Verification items for the finished model (mm, model axes). Face numbers are marked on the shaded views. A direction names the side the tool comes from. Round coordinates to 2 decimals unless told otherwise and drop trailing zeros. Order: outer loops, then holes, each group sorted by start corner. A loop starts at its lowest first (then second) coordinate and runs counter-clockwise, first axis right, second up. Notation, with made-up numbers: (75, 15) -> (122, 15) arc R18 ccw to (122, 39) -> close; hole circle Ø2 at (2, 86.25). An arc over 180 degrees is marked (long way). Return JSON: item names as keys, results as strings. Group by question number.
1) Section check D-D on z = 9. Enter the section's corners in (x, y).
2) Section check A-A on z = 24. Enter the section's corners in (x, y).
3) Section check C-C on y = 20. Enter the section's corners in (x, z), plus the area to 3 significant figures.
4) Tool access check on the marked faces 1 and 2. Record the directions out of +Z, -Z, +X, -X, +Y, -Y that give a thin tool (end or side, any length) a straight path to the whole face; none if there is none.
5) Depth check by flat-ended pin: pin 1 (1 mm diameter, centred on x = -39, y = 18.5, fed in from +Z); pin 2 (7.5 mm diameter, centred on x = -18, y = 40, fed in from -Z); pin 3 (4 mm diameter, centred on x = -7, y = 40, fed in from -Z). Enter the tip coordinate at first touch or a pass-through.
6) Scan lines: L1, parallel to Y at x = -18, z = 3.05; L2, parallel to X at y = 2.5, z = 30.5; L3, parallel to Z at x = -60, y = 13.5. Record each from-to range of solid material in increasing order.
7) Section check B-B on x = -7. Enter the section's corners in (y, z).
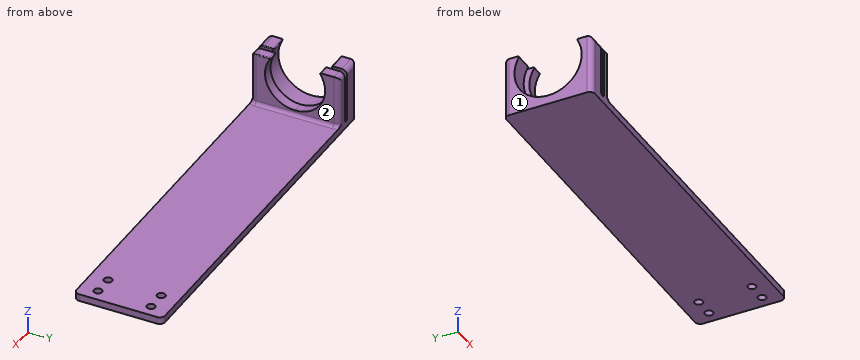
```python
from build123d import *

# Parameters (mm, degrees)
SKETCH_1_W                      = 210
SKETCH_1_H                      = 50
EXTRUDE_1_DEPTH                 = 4
CUT_EXTRUDE_1_REACH             = 217.907
SKETCH_4_R                      = 2.3
CUT_EXTRUDE_1_DIRECTION_2_DEPTH = 216.907387553
EXTRUDE_2_DEPTH                 = 10
EXTRUDE_3_DEPTH                 = 6
FILLET_1_R                      = 3
FILLET_2_R                      = 2
FILLET_3_R                      = 1
FILLET_4_R                      = 0.5


# Some blends are built 0.0001 mm under size
with BuildPart() as part:
    # ｽｹｯﾁ1 → ﾎﾞｽ - 押し出し1 (new body)
    with BuildSketch(Plane.XY):
        with Locations((-105, 25)):
            Rectangle(SKETCH_1_W, SKETCH_1_H)
    extrude(amount=EXTRUDE_1_DEPTH)

    # ｽｹｯﾁ4 → ｶｯﾄ - 押し出し1 (cut, up to next)
    with BuildSketch(Plane.XY.offset(4), mode=Mode.PRIVATE) as cut_extrude_1_sk1:
        with Locations(Location((-7, 40, 0), (0, 0, 180))):
            Circle(SKETCH_4_R)
    cut_extrude_1_tool1 = extrude(cut_extrude_1_sk1.sketch, amount=-CUT_EXTRUDE_1_REACH, mode=Mode.PRIVATE) & part.part
    # ｽｹｯﾁ4 → ｶｯﾄ - 押し出し1 (cut, up to next)
    with BuildSketch(Plane.XY.offset(4), mode=Mode.PRIVATE) as cut_extrude_1_sk2:
        with Locations(Location((-18, 40, 0), (0, 0, 180))):
            Circle(SKETCH_4_R)
    cut_extrude_1_tool2 = extrude(cut_extrude_1_sk2.sketch, amount=-CUT_EXTRUDE_1_REACH, mode=Mode.PRIVATE) & part.part
    # ｽｹｯﾁ4 → ｶｯﾄ - 押し出し1 (cut, up to next)
    with BuildSketch(Plane.XY.offset(4), mode=Mode.PRIVATE) as cut_extrude_1_sk3:
        with Locations(Location((-7, 10, 0), (0, 0, 180))):
            Circle(SKETCH_4_R)
    cut_extrude_1_tool3 = extrude(cut_extrude_1_sk3.sketch, amount=-CUT_EXTRUDE_1_REACH, mode=Mode.PRIVATE) & part.part
    # ｽｹｯﾁ4 → ｶｯﾄ - 押し出し1 (cut, up to next)
    with BuildSketch(Plane.XY.offset(4), mode=Mode.PRIVATE) as cut_extrude_1_sk4:
        with Locations(Location((-18, 10, 0), (0, 0, 180))):
            Circle(SKETCH_4_R)
    cut_extrude_1_tool4 = extrude(cut_extrude_1_sk4.sketch, amount=-CUT_EXTRUDE_1_REACH, mode=Mode.PRIVATE) & part.part
    add(cut_extrude_1_tool1.solids().sort_by_distance((-7, 40, 4))[0], mode=Mode.SUBTRACT)
    add(cut_extrude_1_tool2.solids().sort_by_distance((-18, 40, 4))[0], mode=Mode.SUBTRACT)
    add(cut_extrude_1_tool3.solids().sort_by_distance((-7, 10, 4))[0], mode=Mode.SUBTRACT)
    add(cut_extrude_1_tool4.solids().sort_by_distance((-18, 10, 4))[0], mode=Mode.SUBTRACT)

    # ｽｹｯﾁ4 → ｶｯﾄ - 押し出し1 direction 2 (cut)
    with BuildSketch(Plane.XY.offset(4)):
        with Locations(Location((-7, 40, 0), (0, 0, 180))):
            Circle(SKETCH_4_R)
        with Locations(Location((-18, 40, 0), (0, 0, 180))):
            Circle(SKETCH_4_R)
        with Locations(Location((-7, 10, 0), (0, 0, 180))):
            Circle(SKETCH_4_R)
        with Locations(Location((-18, 10, 0), (0, 0, 180))):
            Circle(SKETCH_4_R)
    extrude(amount=CUT_EXTRUDE_1_DIRECTION_2_DEPTH, mode=Mode.SUBTRACT)

    # ｽｹｯﾁ5 → ﾎﾞｽ - 押し出し2 (add)
    with BuildSketch(Plane.ZY.offset(210)):
        with BuildLine():
            Line((34, 50), (4, 50))
            Line((4, 50), (4, 0))
            Line((4, 0), (34, 0))
            Line((34, 0), (34, 8.844505579))
            ThreePointArc((34, 8.844505579), (5, 25), (34, 41.155494421))
            Line((34, 41.155494421), (34, 50))
        make_face()
    extrude(amount=-EXTRUDE_2_DEPTH)

    # ｽｹｯﾁ6 → ﾎﾞｽ - 押し出し3 (add)
    with BuildSketch(Plane(origin=(-197.7, 0, 0), x_dir=(0, 0, -1), z_dir=(1, 0, 0))):
        with BuildLine():
            Line((-4, 50), (-34, 50))
            Line((-34, 50), (-34, 38.747727085))
            ThreePointArc((-34, 38.747727085), (-16.28637569, 40.149257408), (-7, 25))
            ThreePointArc((-7, 25), (-16.28637569, 9.850742592), (-34, 11.252272915))
            Line((-34, 11.252272915), (-34, 0))
            Line((-34, 0), (-4, 0))
            Line((-4, 0), (-4, 50))
        make_face()
    extrude(amount=EXTRUDE_3_DEPTH)

    # ﾌｨﾚｯﾄ1
    fillet_1_edges = [part.edges().sort_by_distance(p)[0] for p in [
        (-205, 0, 34),
        (-205, 50, 34),
        (-194.7, 0, 34),
        (-191.7, 50, 19),
        (-194.7, 50, 34),
        (-191.7, 0, 19),
        (0, 0, 2),
        (-210, 0, 17),
        (-210, 50, 17),
        (0, 50, 2),
    ]]
    fillet(fillet_1_edges, radius=FILLET_1_R)

    # ﾌｨﾚｯﾄ2
    # the kernel refuses this fillet: 2 mm, written as the material it adds along each edge
    with BuildSketch(Plane(origin=(-191.7, 3, 4), x_dir=(0, 0, 1), z_dir=(0, 1, 0))) as fillet_2_piece_1:
        with BuildLine():
            CenterArc((FILLET_2_R, FILLET_2_R), FILLET_2_R, 180, 90)
            Line((0, FILLET_2_R), (0, 0))
            Line((0, 0), (FILLET_2_R, 0))
        make_face()
    extrude(amount=44)
    with BuildSketch(Plane(origin=(-194.7, 3, 4), x_dir=(-0.9953436464450918, 0.0963899656675329, 0), z_dir=(0.0963899656675329, 0.9953436464450918, 0))) as fillet_2_piece_2_section:
        with BuildLine():
            CenterArc((3 + FILLET_2_R, FILLET_2_R), FILLET_2_R, 180, 90)
            Line((3 + FILLET_2_R, 0), (3, 0))
            Line((3, 0), (3, FILLET_2_R))
        make_face()
    fillet_2_piece_2 = revolve(axis=Axis((-194.7, 3, 4), (0, 0, 1)), revolution_arc=185.531326158, mode=Mode.PRIVATE)
    fillet_2_piece_2 = split(fillet_2_piece_2, bisect_by=Plane(origin=(-192.479113514, 0, 4.573600846), z_dir=(0, 1, 0)), keep=Keep.TOP, mode=Mode.PRIVATE)
    fillet_2_piece_2 = split(fillet_2_piece_2, bisect_by=Plane(origin=(-197.7, 0.779113097, 4.573600846), z_dir=(1, 0, 0)), keep=Keep.TOP, mode=Mode.PRIVATE)
    add(fillet_2_piece_2)
    with BuildSketch(Plane(origin=(-194.7, 47, 4), x_dir=(-0.9953436464450918, -0.09638996566753365, 0), z_dir=(0.09638996566753365, -0.9953436464450918, 0))) as fillet_2_piece_3_section:
        with BuildLine():
            CenterArc((3 + FILLET_2_R, -FILLET_2_R), FILLET_2_R, 90, 90)
            Line((3 + FILLET_2_R, 0), (3, 0))
            Line((3, 0), (3, -FILLET_2_R))
        make_face()
    fillet_2_piece_3 = revolve(axis=Axis((-194.7, 47, 4), (0, 0, -1)), revolution_arc=185.531326158, mode=Mode.PRIVATE)
    fillet_2_piece_3 = split(fillet_2_piece_3, bisect_by=Plane(origin=(-192.479113243, 50, 4.573600331), z_dir=(0, -1, 0)), keep=Keep.TOP, mode=Mode.PRIVATE)
    fillet_2_piece_3 = split(fillet_2_piece_3, bisect_by=Plane(origin=(-197.7, 49.22088673, 4.573600331), z_dir=(1, 0, 0)), keep=Keep.TOP, mode=Mode.PRIVATE)
    add(fillet_2_piece_3)

    # ﾌｨﾚｯﾄ3
    fillet_3_edges = [part.edges().sort_by_distance(p)[0] for p in [
        (-200, 25, 4),
        (-197.7, 25, 4),
    ]]
    fillet(fillet_3_edges, radius=FILLET_3_R - 0.0001)  # a hair under: the kernel refuses the full size

    # ﾌｨﾚｯﾄ4
    fillet_4_edges = [part.edges().sort_by_distance(p)[0] for p in [
        (-192.761853278, 0.71011195, 32.938146722),
        (-200, 5.922252789, 34),
        (-200, 0.878679656, 33.121320344),
        (-200, 0, 17.99995),
        (-199.707136071, 0, 4.292863929),
        (-198.85, 0, 4),
        (-197.992863929, 0, 4.292863929),
        (-197.7, 0, 17.99995),
        (-197.7, 0.878679656, 33.121320344),
        (-194.7, 11.252272915, 34),
        (-194.7, 38.747727085, 34),
        (-191.7, 7.126136458, 34),
        (-197.7, 7.126136458, 34),
        (-205, 8.844505579, 34),
        (-205, 41.155494421, 34),
    ]]
    fillet(fillet_4_edges, radius=FILLET_4_R)


solid = part.part
```
Check result:
{
 "1": {"outline": "(-210, 3) arc R3 ccw to (-207, 0) -> (-200.5, 0) arc R0.5 ccw to (-200, 0.5) -> (-200, 13.34) -> (-210, 13.34) -> close; (-210, 36.66) -> (-200, 36.66) -> (-200, 50) -> (-207, 50) arc R3 ccw to (-210, 47) -> close; (-197.7, 0.5) arc R0.5 ccw to (-197.2, 0) -> (-194.7, 0) arc R3 ccw to (-191.7, 3) -> (-191.7, 17) -> (-197.7, 17) -> close; (-197.7, 33) -> (-191.7, 33) -> (-191.7, 47) arc R3 ccw to (-194.7, 50) -> (-197.7, 50) -> close"},
 "2": {"outline": "(-210, 3) arc R3 ccw to (-207, 0) -> (-200.5, 0) arc R0.5 ccw to (-200, 0.5) -> (-200, 6) -> (-210, 6) -> close; (-210, 44) -> (-200, 44) -> (-200, 50) -> (-207, 50) arc R3 ccw to (-210, 47) -> close; (-197.7, 0.5) arc R0.5 ccw to (-197.2, 0) -> (-194.7, 0) arc R3 ccw to (-191.7, 3) -> (-191.7, 8) -> (-197.7, 8) -> close; (-197.7, 42) -> (-191.7, 42) -> (-191.7, 47) arc R3 ccw to (-194.7, 50) -> (-197.7, 50) -> close"},
 "3": {"outline": "(-210, 0) -> (0, 0) -> (0, 4) -> (-189.7, 4) arc R2 cw to (-191.7, 6) -> (-191.7, 7.75) -> (-197.7, 7.75) -> (-197.7, 5) arc R1 cw to (-198.7, 4) -> (-199, 4) arc R1 cw to (-200, 5) -> (-200, 5.67) -> (-210, 5.67) -> close", "area": "880 mm^2"},
 "4": {"face 1": "+Z, -Z, -X, +Y, -Y", "face 2": "+Z, +X, +Y, -Y"},
 "5": {"pin 1": "z = 4", "pin 2": "z = 0", "pin 3": "through"},
 "6": {"L1": "0 to 7.7, 12.3 to 37.7, 42.3 to 50", "L2": "-209.96 to -200, -197.7 to -191.74", "L3": "0 to 4"},
 "7": {"outline": "(0, 0) -> (7.7, 0) -> (7.7, 4) -> (0, 4) -> close; (12.3, 0) -> (37.7, 0) -> (37.7, 4) -> (12.3, 4) -> close; (42.3, 0) -> (50, 0) -> (50, 4) -> (42.3, 4) -> close"}
}
